CAD build for the part. Positions are in the model's coordinates, mm. Face numbers are marked on the shaded views. A direction names the side the tool comes from. Coordinates: 2 decimals unless noted, no trailing zeros. Loops run counter-clockwise (first coordinate to the right, second up) from the corner with the lowest first, then second, coordinate; pieces in that order, holes last. Notation, with made-up numbers: M 20.5,68.5 L 43.5,68.5 A22 ccw 43.5,97.5 Z; hole C 36,82 d8. An arc over 180 degrees is marked long. Answer as a JSON object with one key per item and string values. Group by question number.
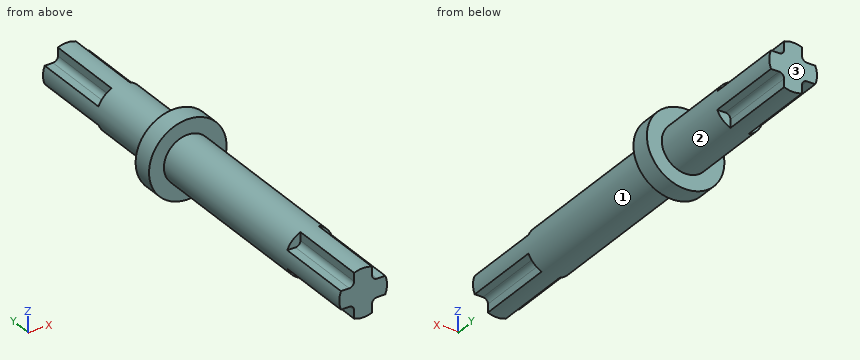
Autodesk Inventor part; units mm, degrees
ref_plane "YZ Plane" through (0, 0, 0) normal (1, 0, 0) x (0, 1, 0)
ref_plane "XZ Plane" through (0, 0, 0) normal (0, 1, 0) x (-1, 0, 0)
ref_plane "XY Plane" through (0, 0, 0) normal (0, 0, 1) x (1, 0, 0)
sketch "Sketch1" plane through (0, 0, 0) normal (0, 1, 0) x (-1, 0, 0)
  line L0 (0.9, 2.4) -> (-0.9, 2.4)
  line L1 (0.9, 2.4) -> (0.9, 1.4)
  line L2 (1.4, 1.4) -> (0.9, 1.4) construction
  line L3 (1.4, 1.4) -> (1.4, 0.9) construction
  arc A0 (0.9, 1.4) -> (1.4, 0.9) centre (1.4, 1.4) ccw
  line L4 (1.4, 0.9) -> (2.4, 0.9)
  line L5 (-0.9, 1.4) -> (-0.9, 2.4)
  arc A1 (-1.4, 0.9) -> (-0.9, 1.4) centre (-1.4, 1.4) ccw
  line L6 (-2.4, 0.9) -> (-1.4, 0.9)
  line L7 (-2.4, 0.9) -> (-2.4, -0.9)
  line L8 (-1.4, -0.9) -> (-2.4, -0.9)
  arc A2 (-0.9, -1.4) -> (-1.4, -0.9) centre (-1.4, -1.4) ccw
  line L9 (-0.9, -2.4) -> (-0.9, -1.4)
  line L10 (-0.9, -2.4) -> (0.9, -2.4)
  line L11 (0.9, -1.4) -> (0.9, -2.4)
  arc A3 (1.4, -0.9) -> (0.9, -1.4) centre (1.4, -1.4) ccw
  line L12 (2.4, -0.9) -> (1.4, -0.9)
  line L13 (2.4, -0.9) -> (2.4, 0.9)
  line L14 (0, 2.4) -> (0, -2.4) construction
  circle A4 centre (0, 0) radius 2.4
  circle A5 centre (0, 0) radius 3.9
  point P0 (0, 0)
  point P1 (0, 0)
  point P2 (-2.4, 0)
  point P3 (2.4, 0)
  point P4 (2.2249, -0.9)
  point P5 (2.2249, 0.9)
  point P6 (0.9, 2.2249)
  point P7 (-0.9, 2.2249)
  point P8 (-2.2249, 0.9)
  point P9 (-2.2249, -0.9)
  point P10 (-0.9, -2.2249)
  point P11 (0.9, -2.2249)
  dimension "d6" = 1.8
  dimension "d7" = 2.4
  dimension "d8" = 1
  dimension "d9" = 0.5
  dimension "d10" = 1
  dimension "d11" = 360
  dimension "d12" = 2.4
  dimension "d13" = 0.9
  dimension "d16" = 4.8
  dimension "d24" = 7.8
extrude "Extrusion2" add sketch "Sketch1" along normal blind 8 contours A4 L1 A0 L4 L12 A3 L11 L9 A2 L8 L6 A1 L5
extrude "Extrusion3" add sketch "Sketch1" along normal blind 18.1 from surface at 8 contours A4 L1 A0 L4 L12 A3 L11 L9 A2 L8 L6 A1 L5 | A4 L4 A0 L1 | L5 A1 L6 A4 | A4 L11 A3 L12 | L8 A2 L9 A4
extrude "Extrusion5" add sketch "Sketch1" along normal blind 2 from surface at 26.1 contours L1 A4 L0 | A4 L5 L0 | A4 L1 A0 L4 L12 A3 L11 L9 A2 L8 L6 A1 L5 | A4 L4 A0 L1 | L5 A1 L6 A4 | L4 L13 A4 | A4 L7 L6 | L13 L12 A4 | A4 L8 L7 | A4 L11 A3 L12 | L8 A2 L9 A4 | L11 L10 A4 | A4 L10 L9 | A5
extrude "Extrusion6" add sketch "Sketch1" along normal blind 8 from surface at 28.1 contours A4 L1 A0 L4 L12 A3 L11 L9 A2 L8 L6 A1 L5 | A4 L4 A0 L1 | L5 A1 L6 A4 | A4 L11 A3 L12 | L8 A2 L9 A4
extrude "Extrusion7" add sketch "Sketch1" along normal blind 8 from surface at 36.1 contours A4 L1 A0 L4 L12 A3 L11 L9 A2 L8 L6 A1 L5
properties part number "diff_gear_holder_2"
Item 1: Slice it at B-B, the plane x = 0. Write the cut outline in (y, z), then the cut area to 3 significant figures.
Item 2: Slice it at C-C, the plane y = 38.5. Write the cut outline in (x, z).
Item 3: Tool access for the marked faces 1, 2 and 3: list every direction of +Z, -Z, +X, -X, +Y, -Y with a clear straight run to the whole face (end or side of a thin tool).
Item 4: Slice it at D-D, the plane y = 13. Write the cut outline in (x, z).
Item 5: Pin check, flat tips, straight feed: pin 1 (0.9 mm diameter, centred on x = -1.5, y = 39.5, fed in from -Z); pin 2 (1.1 mm diameter, centred on x = -1.5, z = 1.5, fed in from +Y); pin 3 (0.9 mm diameter, centred on x = -2, y = 39, fed in from +Z); pin 4 (1.5 mm diameter, centred on y = 28.5, z = -0.5, fed in from -X). Stop position of each tip, or through.
Item 6: Slice it at A-A, the plane z = 0. Write the cut outline in (x, y).
Item 7: Drill centre lines: L1, parallel to Z at x = 2, y = 2; L2, parallel to Y at x = -3, z = 1.75; L3, parallel to Z at x = 0, y = 16.5. Where is each one in solid material? Low to high. Write a range as from..to.
Computed:
{
 "1": {"outline": "M 0,-2.4 L 26.1,-2.4 L 26.1,-3.9 L 28.1,-3.9 L 28.1,-2.4 L 44.1,-2.4 L 44.1,2.4 L 28.1,2.4 L 28.1,3.9 L 26.1,3.9 L 26.1,2.4 L 0,2.4 Z", "area": "218 mm2"},
 "2": {"outline": "M -2.22,-0.9 L -1.4,-0.9 A0.5 cw -0.9,-1.4 L -0.9,-2.22 A2.4 ccw 0.9,-2.22 L 0.9,-1.4 A0.5 cw 1.4,-0.9 L 2.22,-0.9 A2.4 ccw 2.22,0.9 L 1.4,0.9 A0.5 cw 0.9,1.4 L 0.9,2.22 A2.4 ccw -0.9,2.22 L -0.9,1.4 A0.5 cw -1.4,0.9 L -2.22,0.9 A2.4 ccw Z"},
 "3": {"face 1": "-Y", "face 2": "+Y", "face 3": "+Z, -Z, +X, -X, +Y"},
 "4": {"outline": "C 0,0 d4.8"},
 "5": {"pin 1": "z = -1.04", "pin 2": "y = 36.1", "pin 3": "z = 0.9", "pin 4": "x = -3.9"},
 "6": {"outline": "M -3.9,26.1 L -2.4,26.1 L -2.4,0 L 2.4,0 L 2.4,26.1 L 3.9,26.1 L 3.9,28.1 L 2.4,28.1 L 2.4,44.1 L -2.4,44.1 L -2.4,28.1 L -3.9,28.1 Z"},
 "7": {"L1": "-0.9..0.9", "L2": "26.1..28.1", "L3": "-2.4..2.4"}
}
